For this review, take the finished solid that the model builds, in its own axes (mm). Face numbers are marked on the shaded views. A direction names the side the tool comes from. Give positions to 0.01 mm unless a question says otherwise; leave off trailing zeros. Write each loop counter-clockwise with the first axis right and the second up, starting at its lowest first coordinate (ties: lowest second). Pieces come first, ordered by that corner, then holes.
Q1. For line 1 (X direction, y = 13.5, z = 33.5); line 2 (X direction, y = 5, z = 17); line 3 (Z direction, x = -26, y = 12.5), list the stretches that pass through material, from the lowest coordinate up.
Q2. We need section D-D (x = -35). Write out the cut boundary in (y, z), then the cut area to 3 significant figures.
Q3. We need section B-B (y = 10.5). Write out the cut boundary in (x, z) (3 decimals), then the cut area to 3 significant figures.
Q4. We need section C-C (x = -8.56). Write out the cut boundary in (y, z) (3 decimals).
Q5. Mouldability with a two-part tool opening along Z and no side actions: class the marked faces 4, 5, 6 and 7 as released by +Z, released by -Z, zero draft, split by the parting line, or undercut.
Q6. We need section A-A (z = -23). Write out the cut boundary in (x, y).
Q7. Machinability: for the marked faces 1, 2 and 3, which of the approach directions +Z, -Z, +X, -X, +Y, -Y give a long, thin tool a straight path to every point of the face, cutting with its end or side? Answer none if there is none.
Q8. Insertion check: P1, Ø2.5, axis at x = -35, y = -4, coming from the -Z side; P2, Ø0.6, axis at y = -5.5, z = -53.5, coming from the -X side; P3, Ø9, axis at x = -34.5, z = -49.5, coming from the -Y side. Each pin has a flat end and moves straight along its axis. Give the tip position at first contact, or say it passes through.
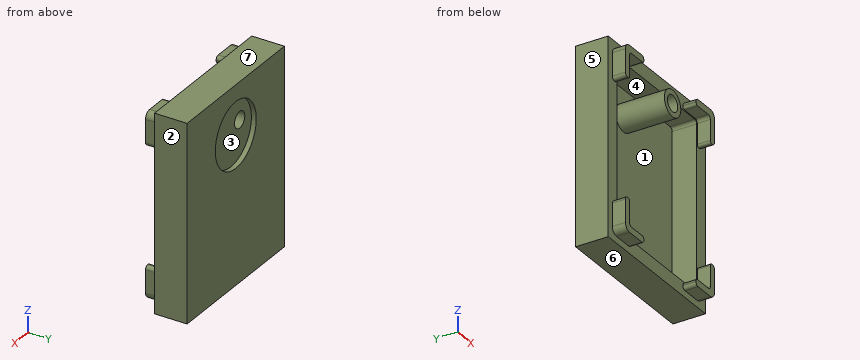
```python
from build123d import *

# Parameters (mm, degrees)
SKETCH2_W                                  = 95
SKETCH2_H                                  = 120
TOP_PLATE_DEPTH                            = 20
FRICTION_CLIP_DEPTH                        = 8
F_4_CLIPS_AT_THE_SECOND_PLANE_COPY_1_DEPTH = 8
CUT_EXTRUDE1_DEPTH                         = 15
SKETCH5_R                                  = 5
SNOOZE_HOLE_DEPTH                          = 29
SKETCH6_R                                  = 8
SKETCH6_R_2                                = 5
SNOOZE_HOLE_SUPPORT_DEPTH                  = 15
SNOOZE_HOLE_SUPPORT_DEPTH_BACK             = 15
SKETCH9_R                                  = 20
LAKE_INLAY_DEPTH                           = 3


with BuildPart() as part:
    # Sketch2 → top plate (new body)
    with BuildSketch(Plane(origin=(0, 0, 0), x_dir=(1, 0, 0), z_dir=(0, 1, 0))):
        Rectangle(SKETCH2_W, SKETCH2_H)
    extrude(amount=TOP_PLATE_DEPTH)

    # Sketch3 → friction clip (add)
    with BuildSketch(Plane.XZ):
        with BuildLine():
            Line((-37.45, 51.95), (-26.95, 51.95))
            ThreePointArc((-26.95, 51.95), (-25.889339828, 52.389339828), (-25.45, 53.45))
            Line((-25.45, 53.45), (-25.45, 53.95))
            ThreePointArc((-25.45, 53.95), (-26.035786438, 55.364213562), (-27.45, 55.95))
            Line((-27.45, 55.95), (-39.45, 55.95))
            ThreePointArc((-39.45, 55.95), (-42.278427125, 54.778427125), (-43.45, 51.95))
            Line((-43.45, 51.95), (-43.45, 37.95))
            ThreePointArc((-43.45, 37.95), (-42.864213562, 36.535786438), (-41.45, 35.95))
            Line((-41.45, 35.95), (-40.95, 35.95))
            ThreePointArc((-40.95, 35.95), (-39.889339828, 36.389339828), (-39.45, 37.45))
            Line((-39.45, 37.45), (-39.45, 49.95))
            ThreePointArc((-39.45, 49.95), (-38.864213562, 51.364213562), (-37.45, 51.95))
        make_face()
    friction_clip = extrude(amount=FRICTION_CLIP_DEPTH)

    # 4 clips: friction clip across plane
    add(friction_clip.mirror(Plane.XY))

    # 4 clips at the second plane: friction clip across plane
    add(friction_clip.mirror(Plane(origin=(0, 0, 0), x_dir=(0, 0, 1), z_dir=(1, 0, 0))))

    # 4 clips at the second plane copy 1 sketc → 4 clips at the second plane copy 1 (add)
    with BuildSketch(Plane(origin=(0, 0, 0), x_dir=(-1, 0, 0), z_dir=(0, -1, 0))):
        with BuildLine():
            Line((-37.45, 51.95), (-26.95, 51.95))
            ThreePointArc((-26.95, 51.95), (-25.889339828, 52.389339828), (-25.45, 53.45))
            Line((-25.45, 53.45), (-25.45, 53.95))
            ThreePointArc((-25.45, 53.95), (-26.035786438, 55.364213562), (-27.45, 55.95))
            Line((-27.45, 55.95), (-39.45, 55.95))
            ThreePointArc((-39.45, 55.95), (-42.278427125, 54.778427125), (-43.45, 51.95))
            Line((-43.45, 51.95), (-43.45, 37.95))
            ThreePointArc((-43.45, 37.95), (-42.864213562, 36.535786438), (-41.45, 35.95))
            Line((-41.45, 35.95), (-40.95, 35.95))
            ThreePointArc((-40.95, 35.95), (-39.889339828, 36.389339828), (-39.45, 37.45))
            Line((-39.45, 37.45), (-39.45, 49.95))
            ThreePointArc((-39.45, 49.95), (-38.864213562, 51.364213562), (-37.45, 51.95))
        make_face()
    extrude(amount=F_4_CLIPS_AT_THE_SECOND_PLANE_COPY_1_DEPTH)

    # Sketch8 → Cut-Extrude1 (cut)
    with BuildSketch(Plane.XZ):
        with BuildLine():
            Line((-36.864213562, -51.364213562), (36.864213562, -51.364213562))
            ThreePointArc((36.864213562, -51.364213562), (38.278427125, -50.778427125), (38.864213562, -49.364213562))
            Line((38.864213562, -49.364213562), (38.864213562, 49.364213562))
            ThreePointArc((38.864213562, 49.364213562), (38.278427125, 50.778427125), (36.864213562, 51.364213562))
            Line((36.864213562, 51.364213562), (-36.864213562, 51.364213562))
            ThreePointArc((-36.864213562, 51.364213562), (-38.278427125, 50.778427125), (-38.864213562, 49.364213562))
            Line((-38.864213562, 49.364213562), (-38.864213562, -49.364213562))
            ThreePointArc((-38.864213562, -49.364213562), (-38.278427125, -50.778427125), (-36.864213562, -51.364213562))
        make_face()
    extrude(amount=-CUT_EXTRUDE1_DEPTH, mode=Mode.SUBTRACT)

    # Sketch5 → snooze hole (cut, through all)
    with BuildSketch(Plane(origin=(0, 20, 0), x_dir=(1, 0, 0), z_dir=(0, 1, 0))):
        with Locations((-8.56, -34.015)):
            Circle(SKETCH5_R)
    extrude(amount=-SNOOZE_HOLE_DEPTH, mode=Mode.SUBTRACT)

    # Sketch6 → snooze hole support (add, two sides)
    with BuildSketch(Plane.XZ) as snooze_hole_support_sk:
        with Locations((-8.56, 34.015)):
            Circle(SKETCH6_R)
        with Locations((-8.56, 34.015)):
            Circle(SKETCH6_R_2, mode=Mode.SUBTRACT)
    extrude(amount=SNOOZE_HOLE_SUPPORT_DEPTH)
    extrude(snooze_hole_support_sk.sketch, amount=-SNOOZE_HOLE_SUPPORT_DEPTH_BACK)

    # Sketch9 → lake inlay (cut)
    with BuildSketch(Plane(origin=(0, 20, 0), x_dir=(1, 0, 0), z_dir=(0, 1, 0))):
        with Locations((0, -30)):
            Circle(SKETCH9_R)
    extrude(amount=-LAKE_INLAY_DEPTH, mode=Mode.SUBTRACT)


solid = part.part
```
Computed:
1. line 1: x = -47.5 to -38.86, -16.54 to -13.53, -3.59 to -0.58, 38.86 to 47.5
1. line 2: x = -47.5 to -38.86, 38.86 to 47.5
1. line 3: z = -60 to -51.36, 51.36 to 60
2. outline: (-8, -55.95) - (0, -55.95) - (0, -60) - (20, -60) - (20, 60) - (0, 60) - (0, 55.95) - (-8, 55.95) - (-8, 51.95) - (0, 51.95) - (0, 51.36) - (15, 51.36) - (15, -51.36) - (0, -51.36) - (0, -51.95) - (-8, -51.95) - close
2. area: 923 mm2
3. outline: (-47.5, -60) - (47.5, -60) - (47.5, 60) - (-47.5, 60) - close; circle Ø16 at (-8.56, 34.015); hole (-38.864, -49.364) arc R2 ccw to (-36.864, -51.364) - (36.864, -51.364) arc R2 ccw to (38.864, -49.364) - (38.864, 49.364) arc R2 ccw to (36.864, 51.364) - (-36.864, 51.364) arc R2 ccw to (-38.864, 49.364) - close; hole circle Ø10 at (-8.56, 34.015)
3. area: 3,540 mm2
4. outline: (-15, 26.015) - (15, 26.015) - (15, -51.364) - (0, -51.364) - (0, -60) - (20, -60) - (20, 11.924) - (17, 11.924) - (17, 29.015) - (-15, 29.015) - close; (-15, 39.015) - (17, 39.015) - (17, 48.076) - (20, 48.076) - (20, 60) - (0, 60) - (0, 51.364) - (15, 51.364) - (15, 42.015) - (-15, 42.015) - close
5. face 4: undercut
5. face 5: zero draft
5. face 6: released by -Z
5. face 7: released by +Z
6. outline: (-47.5, 0) - (-38.86, 0) - (-38.86, 15) - (38.86, 15) - (38.86, 0) - (47.5, 0) - (47.5, 20) - (-47.5, 20) - close
7. face 1: -Y
7. face 2: +Z, -Z, +X, +Y, -Y
7. face 3: +Y
8. P1: stops at z = -55.95
8. P2: stops at x = -43.25
8. P3: stops at y = -8
